Geometry: final body of the model. Coordinates: model frame, mm. Give positions to 0.01 mm unless a question says otherwise; leave off trailing zeros. Write each loop counter-clockwise with the first axis right and the second up, starting at its lowest first coordinate (ties: lowest second). Pieces come first, ordered by that corner, then holes. Notation, with made-up numbers: M 77.5,21.5 L 102.5,21.5 A20 cw 102.5,51.5 Z; hole C 67,14 d9. An arc over 180 degrees is marked long. One line per question, with ' | ' between items.
from build123d import *

# Parameters (mm, degrees)
BOSS_EXTRUDE1_DEPTH = 6
SKETCH9_R           = 7.975
CUT_EXTRUDE5_DEPTH  = 5.1
SKETCH10_R          = 2.55
CUT_EXTRUDE6_DEPTH  = 1.9
SKETCH11_R          = 2.55
CUT_EXTRUDE7_DEPTH  = 7
CHAMFER1_SIZE       = 0.5


with BuildPart() as part:
    # Sketch4 → Boss-Extrude1 (new body)
    with BuildSketch(Plane.XY):
        with BuildLine():
            Line((-60, 15), (60, 15))
            ThreePointArc((60, 15), (75, 0), (60, -15))
            Line((60, -15), (-60, -15))
            ThreePointArc((-60, -15), (-75, 0), (-60, 15))
        make_face()
    extrude(amount=BOSS_EXTRUDE1_DEPTH)

    # Sketch9 → Cut-Extrude5 (cut)
    with BuildSketch(Plane(origin=(0, 0, 0), x_dir=(-1, 0, 0), z_dir=(0, 0, -1))):
        with Locations((-60, 0)):
            Circle(SKETCH9_R)
    extrude(amount=-CUT_EXTRUDE5_DEPTH, mode=Mode.SUBTRACT)

    # Sketch10 → Cut-Extrude6 (cut, through all)
    with BuildSketch(Plane(origin=(0, 0, 5.1), x_dir=(-1, 0, 0), z_dir=(0, 0, -1))):
        with Locations((-60, 0)):
            Circle(SKETCH10_R)
    extrude(amount=-CUT_EXTRUDE6_DEPTH, mode=Mode.SUBTRACT)

    # Sketch11 → Cut-Extrude7 (cut, through all)
    with BuildSketch(Plane(origin=(0, 0, 0), x_dir=(-1, 0, 0), z_dir=(0, 0, -1))):
        with Locations((60, 0)):
            Circle(SKETCH11_R)
    extrude(amount=-CUT_EXTRUDE7_DEPTH, mode=Mode.SUBTRACT)

    # Chamfer1
    chamfer1_edges = [part.edges().sort_by_distance(p)[0] for p in [
        (67.975, 0, 0),
    ]]
    chamfer(chamfer1_edges, length=CHAMFER1_SIZE)


solid = part.part
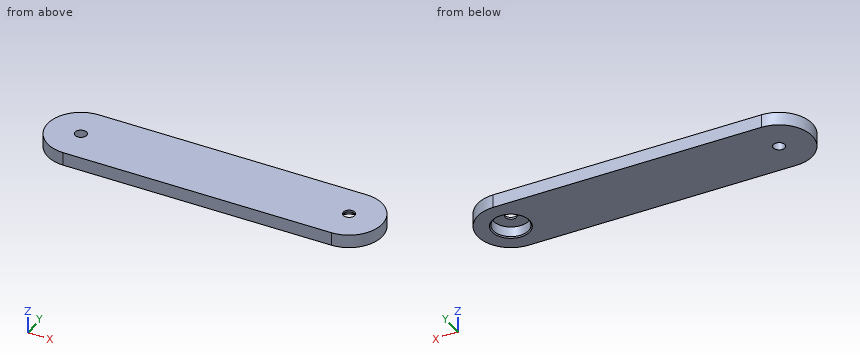
(1) Cut plane A-A, the plane z = 4.15. Return loops of the section in (x, y) (3 decimals), then the cut area to 3 significant figures.
Working result:
outline: M -60,-15 L 60,-15 A15 ccw 60,15 L -60,15 A15 ccw Z; hole C -60,0 d5.1; hole C 60,0 d15.95 | area: 4,090 mm^2
(2) Cut plane B-B, the plane y = -10. Return loops of the section in (x, z), then the cut area to 3 significant figures.
Working result:
outline: M -71.18,0 L 71.18,0 L 71.18,6 L -71.18,6 Z | area: 854 mm^2
(3) Material intervals for L1, parallel to Y at x = -60, z = 3.3; L2, parallel to X at y = 3.5, z = 4.95; L3, parallel to Y at x = 55, z = 3.25, sorted ascending. Write a range as [from, to].
Working result:
L1: y = [-15, -2.55], [2.55, 15] | L2: x = [-74.59, 52.83], [67.17, 74.59] | L3: y = [-15, -6.21], [6.21, 15]
(4) Cut plane C-C, the plane y = 11. Return loops of the section in (x, z).
Working result:
outline: M -70.2,0 L 70.2,0 L 70.2,6 L -70.2,6 Z
(5) First-contact query: P1, Ø8, axis at x = 60, y = 0, coming from the -Z side. Flat tip, straight axial feed; report the tip coordinate or a pass-through.
Working result:
P1: stops at z = 5.1
